Check sheet for the modelled part. Datum: model origin and axes. Units: mm. A direction names the side the tool comes from. Give positions to 0.01 mm unless a question says otherwise; leave off trailing zeros. Write each loop counter-clockwise with the first axis right and the second up, starting at its lowest first coordinate (ties: lowest second). Pieces come first, ordered by that corner, then holes. Notation, with made-up numbers: (71, -2.75) - (106, -2.75) arc R21 ccw to (106, 30.25) - close; hole circle Ø6 at (-22, 7). An arc over 180 degrees is marked (long way). Return JSON: item names as keys, results as strings. Group by question number.
```python
from build123d import *

# Parameters (mm, degrees)
BOSS_EXTRUDE1_DEPTH = 15


with BuildPart() as part:
    # Sketch1 → Boss-Extrude1 (new body)
    with BuildSketch(Plane(origin=(0, 0, 0), x_dir=(1, 0, 0), z_dir=(0, 1, 0))):
        with BuildLine():
            ThreePointArc((-4.666988449, -23.116263327), (53.611641171, 3.020021854), (-4.666988449, 29.156307034))
            Line((-4.666988449, 29.156307034), (-29.36028846, 7.162891325))
            ThreePointArc((-29.36028846, 7.162891325), (-32.406824983, 5.804125188), (-35.678317621, 6.456019442))
            Line((-35.678317621, 6.456019442), (-45.569853208, 11.92154995))
            ThreePointArc((-45.569853208, 11.92154995), (-60.658358829, 3.020021854), (-45.569853208, -5.881506243))
            Line((-45.569853208, -5.881506243), (-35.678317621, -0.415975734))
            ThreePointArc((-35.678317621, -0.415975734), (-32.406824983, 0.235918519), (-29.36028846, -1.122847618))
            Line((-29.36028846, -1.122847618), (-4.666988449, -23.116263327))
        make_face()
        with BuildLine():
            ThreePointArc((-46.053482079, -5.006233077), (-59.658358829, 3.020021854), (-46.053482079, 11.046276784))
            Line((-46.053482079, 11.046276784), (-36.161946493, 5.580746276))
            ThreePointArc((-36.161946493, 5.580746276), (-32.295637011, 4.810325795), (-28.695184757, 6.41614032))
            Line((-28.695184757, 6.41614032), (-4.001884745, 28.409556029))
            ThreePointArc((-4.001884745, 28.409556029), (52.611641171, 3.020021854), (-4.001884745, -22.369512322))
            Line((-4.001884745, -22.369512322), (-28.695184757, -0.376096613))
            ThreePointArc((-28.695184757, -0.376096613), (-32.295637011, 1.229717913), (-36.161946493, 0.459297432))
            Line((-36.161946493, 0.459297432), (-46.053482079, -5.006233077))
        make_face(mode=Mode.SUBTRACT)
    extrude(amount=BOSS_EXTRUDE1_DEPTH)


solid = part.part
```
Item 1: Material ranges on line 1 along X through (y, z) = (10, 1); line 2 along X through (y, z) = (11.25, -3); line 3 along X through (y, z) = (14.5, -3.5), recorded low to high. Write a range as from..to.
Item 2: Depth check by flat-ended pin: pin 1 (2 mm diameter, centred on y = 5.5, z = 2, fed in from -X); pin 2 (3 mm diameter, centred on x = 34.5, y = 11, fed in from +Z); pin 3 (3 mm diameter, centred on x = 2, y = 10, fed in from -Z); pin 4 (12 mm diameter, centred on x = 39, z = -24, fed in from -Y). Enter the tip coordinate at first touch or a pass-through.
Item 3: Section check A-A on x = -50.5. Record the cut outline in (y, z), plus the area to 3 significant figures.
Item 4: Section check C-C on z = 18. Record the cut outline in (x, y), plus the area to 3 significant figures.
Item 5: Access from +Z, -Z, +X, -X, +Y, -Y to the whole of each face (thin tool, end or side, straight path). Record for faces 4 (the face through (-17.186, 7.395, 11.966)), 5 (the face through (-12.3, 15, -21.3)), 6 (the face through (-32.4, 7.4, -4.8)), 7 (the face through (-16.841, 7.395, -18.314)).
Item 6: Section check B-B on y = 3.75. Record the cut outline in (x, z).
Item 7: Mould release check, pull along X, two halves, no side actions. Record for faces 1 (the face through (-59.654, 7.395, -2.754)), 2 (the face through (53.594, 7.395, -1.894)), 3 (the face through (-12.3, 0, -21.3)): +X half, -X half, draft (parallel to the pull), parting line (faces both ways), or undercut.
Reply:
{
 "1": {"line 1": "-59.83..-58.73, -38.8..-36.74, -29.5..-27.99, 52.37..53.38", "line 2": "-60.66..-59.66, 52.61..53.61", "line 3": "-60.65..-59.65, 52.61..53.61"},
 "2": {"pin 1": "x = -59.83", "pin 2": "z = 28.89", "pin 3": "z = -34.59", "pin 4": "y = 0"},
 "3": {"outline": "(0, -13.19) - (15, -13.19) - (15, -12.19) - (0, -12.19) - close; (0, 6.15) - (15, 6.15) - (15, 7.15) - (0, 7.15) - close", "area": "30.0 mm²"},
 "4": {"outline": "(-10.41, 0) - (-8.91, 0) - (-8.91, 15) - (-10.41, 15) - close; (45.34, 0) - (46.6, 0) - (46.6, 15) - (45.34, 15) - close", "area": "41.5 mm²"},
 "5": {"face 4": "+Z, +Y, -Y", "face 5": "+Z, -Z, +X, -X, +Y", "face 6": "+Y, -Y", "face 7": "-Z, +Y, -Y"},
 "6": {"outline": "(-45.57, -11.92) - (-35.68, -6.46) arc R5.5 cw to (-29.36, -7.16) - (-4.67, -29.16) arc R35 ccw (long way) to (-4.67, 23.12) - (-29.36, 1.12) arc R5.5 cw to (-35.68, 0.42) - (-45.57, 5.88) arc R10.17 ccw (long way) to start; hole (-46.05, -11.05) - (-36.16, -5.58) arc R6.5 cw to (-28.7, -6.42) - (-4, -28.41) arc R34 ccw (long way) to (-4, 22.37) - (-28.7, 0.38) arc R6.5 cw to (-36.16, -0.46) - (-46.05, 5.01) arc R9.17 ccw (long way) to start"},
 "7": {"face 1": "undercut", "face 2": "parting line", "face 3": "draft"}
}
